```python
from build123d import *

# Parameters (mm, degrees)
PAD_DEPTH       = 14
POCKET_DEPTH    = 14.001
POCKET001_DEPTH = 3
SKETCH007_R     = 1.85
POCKET002_DEPTH = 21.001
SKETCH008_R     = 1.8
POCKET003_DEPTH = 5
SKETCH009_W     = 32
SKETCH009_H     = 5
PAD001_DEPTH    = 5
FILLET_R        = 2


with BuildPart() as part:
    # Sketch → Pad (new body)
    with BuildSketch(Plane.XY):
        Polygon((-8, 30), (8, 30), (8, 5), (16, 5), (16, 0), (-16, 0), (-16, 5), (-8, 5), align=None)
    extrude(amount=PAD_DEPTH)

    # Sketch002 → Pocket (cut, through all)
    with BuildSketch(Plane.XY.offset(14)):
        with BuildLine():
            ThreePointArc((-5.012819, 18.154908), (-7.83109, 12.138463), (-5.012819, 6.122018))
            Line((-5.012819, 5), (-5.012819, 6.122018))
            Line((-8.968158, 5), (-5.012819, 5))
            Line((-8.890375, 30.926365), (-8.968158, 5))
            Line((-7.922217, 30.944389), (-8.890375, 30.926365))
            Line((-7.922217, 19), (-7.922217, 30.944389))
            Line((-5.012819, 19), (-7.922217, 19))
            Line((-5.012819, 18.154908), (-5.012819, 19))
        make_face()
        with BuildLine():
            Line((5, 31), (5, 18))
            ThreePointArc((5, 6.276926), (7.670247, 12.138463), (5, 18))
            Line((5, 6.276926), (5, 5))
            Line((10, 5), (5, 5))
            Line((10, 31), (10, 5))
            Line((5, 31), (10, 31))
        make_face()
        with BuildLine():
            ThreePointArc((-2.521136, 17.36186), (-0.003033, 6.338464), (2.526597, 17.35922))
            Line((2.526597, 31), (2.526597, 17.35922))
            Line((-2.521136, 31), (2.526597, 31))
            Line((-2.521136, 17.36186), (-2.521136, 31))
        make_face()
    extrude(amount=-POCKET_DEPTH, mode=Mode.SUBTRACT)

    # Sketch006 → Pocket001 (cut)
    with BuildSketch(Plane(origin=(-7.922217, 0, 0), x_dir=(0, -1, 0), z_dir=(-1, 0, 0))):
        Polygon((-21.086217, 5.037009), (-21.086217, 8.962991), (-24.486217, 10.925982), (-27.886217, 8.962991), (-27.886217, 5.037009), (-24.486217, 3.074018), align=None)
    extrude(amount=-POCKET001_DEPTH, mode=Mode.SUBTRACT)

    # Sketch007 → Pocket002 (cut, through all)
    with BuildSketch(Plane.YZ.offset(5)):
        with Locations((24.472246, 7)):
            Circle(SKETCH007_R)
    extrude(amount=-POCKET002_DEPTH, mode=Mode.SUBTRACT)

    # Sketch008 → Pocket003 (cut)
    with BuildSketch(Plane.XZ):
        with Locations((-12, 5)):
            Circle(SKETCH008_R)
        with Locations((12, 5)):
            Circle(SKETCH008_R)
    extrude(amount=-POCKET003_DEPTH, mode=Mode.SUBTRACT)

    # Sketch009 → Pad001 (new body)
    with BuildSketch(Plane.XZ):
        with Locations((0, 11.5)):
            Rectangle(SKETCH009_W, SKETCH009_H)
    extrude(amount=PAD001_DEPTH)

    # Fillet
    fillet_edges = [part.edges().sort_by_distance(p)[0] for p in [
        (-16, -5, 11.5),
        (16, -5, 11.5),
        (16, 5, 7),
        (5, 30, 7),
        (-16, 5, 7),
        (-7.922217, 30, 7),
        (0, 0, 0),
        (-16, 0, 14),
        (0, -5, 14),
        (16, 0, 14),
        (16, 2.5, 0),
        (-16, 2.5, 0),
        (-7.922217, 24.5, 0),
        (-7.922217, 24.5, 14),
        (-7.922217, 19, 7),
    ]]
    fillet(fillet_edges, radius=FILLET_R)


solid = part.part
```
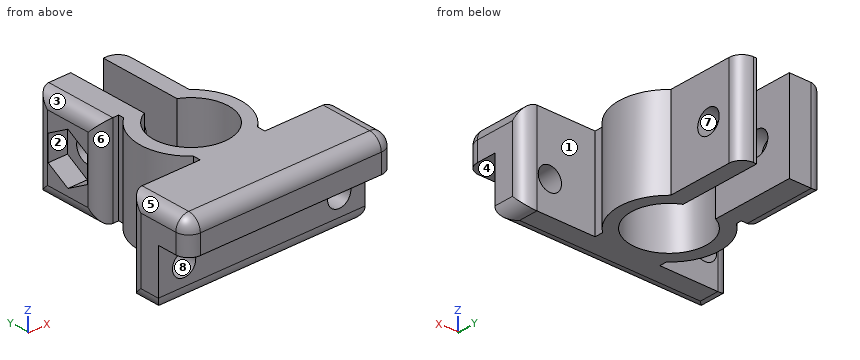
Input: part model. Units: mm. Frame: model coordinates. Face numbers are marked on the shaded views. A direction names the side the tool comes from. Give positions to 0.01 mm unless a question says otherwise; leave off trailing zeros. Order: outer loops, then holes, each group sorted by start corner. A loop starts at its lowest first (then second) coordinate and runs counter-clockwise, first axis right, second up. Notation, with made-up numbers: (-24.75, 20) - (11.25, 20) arc R6 ccw to (11.25, 29) - close; hole circle Ø10 at (30.25, 88). An arc over 180 degrees is marked (long way). Use a Markdown table: item, result.
(1) Section query A-A (x = -12). Output: boundary loops of the cut face in (y, z), then the cut area to 3 significant figures.
Computed values:
| item | result |
|---|---|
| outline | (-5, 9) - (0, 9) - (0, 6.8) - (5, 6.8) - (5, 14) - (-3, 14) arc R2 ccw to (-5, 12) - close; (0, 2) arc R2 ccw to (2, 0) - (5, 0) - (5, 3.2) - (0, 3.2) - close |
| area | 75.3 mm2 |
(2) Section query B-B (x = -3). Output: boundary loops of the cut face in (y, z), then the cut area to 3 significant figures.
Computed values:
| item | result |
|---|---|
| outline | (-5, 9) - (0, 9) - (0, 2) arc R2 ccw to (2, 0) - (7.17, 0) - (7.17, 14) - (-3, 14) arc R2 ccw to (-5, 12) - close; (17.1, 0) - (30, 0) - (30, 14) - (17.1, 14) - close; hole circle Ø3.7 at (24.47, 7) |
| area | 294 mm2 |
(3) Section query D-D (z = 8). State how many separate pieces and enclosed holes the cut face has, then the cut area to 3 significant figures.
Computed values:
| item | result |
|---|---|
| separate pieces | 3 |
| enclosed holes | 0 |
| area | 280 mm2 |
(4) Draft query along Z for the marked faces 5, 6, 7 and 8. Return one class per face: released by +Z, released by -Z, zero draft, split by the parting line, or undercut.
Computed values:
| item | result |
|---|---|
| face 5 | released by +Z |
| face 6 | zero draft |
| face 7 | undercut |
| face 8 | undercut |
(5) Line query: line 1 (X direction, y = 24, z = 3); line 2 (Z direction, x = 12, y = 3); line 3 (Y direction, x = -6.5, z = 3.5). Output: solid intervals per line, ascending. Write a range as from..to.
Computed values:
| item | result |
|---|---|
| line 1 | x = -7.92..-2.52, 2.53..5 |
| line 2 | z = 0..3.2, 6.8..14 |
| line 3 | y = 0..5, 7.77..16.51, 19.09..23.75, 25.22..29.91 |
(6) Pin query (flat end, axial travel): pin 1 (4 mm diameter, centred on y = 24, z = 3.5, fed in from -X); pin 2 (1 mm diameter, centred on x = -5.5, z = 4.5, fed in from -Y); pin 3 (4 mm diameter, centred on x = 2.5, y = -3.5, fed in from -Z). Return the tip coordinate at first contact, or that it passes through.
Computed values:
| item | result |
|---|---|
| pin 1 | stops at x = -7.92 |
| pin 2 | stops at y = 0 |
| pin 3 | stops at z = 9 |
(7) Section query C-C (y = 15). Output: boundary loops of the cut face in (x, z), then the cut area to 3 significant figures.
Computed values:
| item | result |
|---|---|
| outline | (-7.29, 0) - (-5.04, 0) - (-5.04, 14) - (-7.29, 14) - close; (5.04, 0) - (7.12, 0) - (7.12, 14) - (5.04, 14) - close |
| area | 60.5 mm2 |
(8) Access query for the marked faces 1, 2, 3 and 4. Directions: +Z, -Z, +X, -X, +Y, -Y. A direction counts if a zero-diameter tool reaches every point of the face in a straight line with its end or side. Return the directions, or none.
Computed values:
| item | result |
|---|---|
| face 1 | +Z, -Z, +X |
| face 2 | -X |
| face 3 | +Z, -X, +Y |
| face 4 | -Z, +X, -X, -Y |
